Input: part model. Units: mm. Frame: model coordinates. Face numbers are marked on the shaded views. A direction names the side the tool comes from. Give positions to 0.01 mm unless a question says otherwise; leave off trailing zeros. Write each loop counter-clockwise with the first axis right and the second up, starting at its lowest first coordinate (ties: lowest second). Pieces come first, ordered by that corner, then holes. Notation, with made-up numbers: (18.5, -21.5) -> (49.5, -21.5) arc R35 cw to (49.5, 10.5) -> close; hole circle Ø11 at (34, 36.25). An arc over 180 degrees is marked (long way). Return JSON: item names as keys, results as strings. Group by question number.
Item 1: Mould query, pull axis Z, two halves, no side actions, for the marked faces 1, 2 and 3. Classes: released by +Z, released by -Z, zero draft, split by the parting line, or undercut.
Item 2: Line query: line 1 (Z direction, x = 76.75, y = 0); line 2 (Z direction, x = 15.5, y = -12); line 3 (Y direction, x = 15, z = -17). Output: solid intervals per line, ascending. Write a range as [from, to].
Item 3: Section C-C, the plane x = 24. Return loops of the section in (y, z).
Item 4: Set-up query: the marked faces 4 and 5. Return all of +Z, -Z, +X, -X, +Y, -Y with unobstructed straight access to the full face (end or side cutting, diameter ignored); none if empty.
Item 5: Section B-B, the plane x = 80.5. Return loops of the section in (y, z), then the cut area to 3 significant figures.
Item 6: Pin query (flat end, axial travel): P1, Ø4, axis at x = -5.5, z = -20.5, coming from the -Y side; P2, Ø5, axis at x = 25, y = -19.5, coming from the +Z side; P3, Ø10, axis at y = 18, z = 1.5, coming from the +X side (3 decimals); P4, Ø3, axis at x = 51, z = -13, coming from the +Y side. Return the tip coordinate at first contact, or that it passes through.
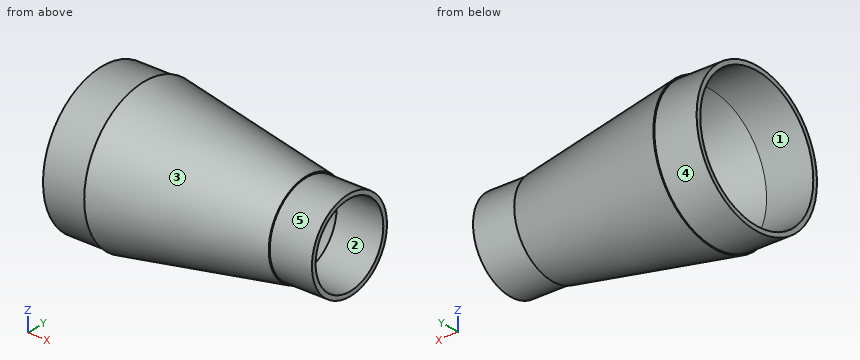
from build123d import *

# Parameters (mm, degrees)
F2_R     = 20.7899
F0_R     = 33.02
F4_R     = 32.4866
F5_DEPTH = 19.05
F6_R     = 20.2565
F7_DEPTH = 19.05
F8_T     = -2.0066


with BuildPart() as f3:
    # F2 (on offset) → F3 section 0
    with BuildSketch(Plane.YZ.offset(73.025)):
        Circle(F2_R)
    # F0 (on Right) → F3 section 1
    with BuildSketch(Plane.YZ):
        Circle(F0_R)
    loft()

    # F4 (on face) → F5 (join)
    with BuildSketch(Plane(origin=(0, 0, 0), x_dir=(0, -1, 0), z_dir=(-1, 0, 0))):
        Circle(F4_R)
    extrude(amount=F5_DEPTH)

    # F6 (on face) → F7 (join)
    with BuildSketch(Plane.YZ.offset(73.025)):
        Circle(F6_R)
    extrude(amount=F7_DEPTH)

    # F8
    f8_openings = [f3.faces().sort_by_distance(p)[0] for p in [
        (92.075, 0, 0),
        (-19.05, 0, 0),
    ]]
    offset(amount=F8_T, openings=f8_openings, kind=Kind.INTERSECTION)


solid = f3.part
Answer below:
{
 "1": {"face 1": "undercut", "face 2": "undercut", "face 3": "split by the parting line"},
 "2": {"line 1": "z = [-20.26, -18.25], [18.25, 20.26]", "line 2": "z = [-27.96, -25.73], [25.73, 27.96]", "line 3": "y = [-25.33, -22.84], [22.84, 25.33]"},
 "3": {"outline": "circle Ø58 at (0, 0); hole circle Ø53.93 at (0, 0)"},
 "4": {"face 4": "-X", "face 5": "+X"},
 "5": {"outline": "circle Ø40.51 at (0, 0); hole circle Ø36.5 at (0, 0)", "area": "243 mm2"},
 "6": {"P1": "stops at y = -26.7", "P2": "stops at z = 23.36", "P3": "stops at x = 92.075", "P4": "stops at y = 21.66"}
}
